```python
from build123d import *

# Parameters (mm, degrees)
BOSS_EXTRUDE1_DEPTH = 5.08
SKETCH4_R           = 104.775
CUT_EXTRUDE1_DEPTH  = 50.8
SKETCH5_R           = 3.175
CUT_EXTRUDE2_DEPTH  = 5.08
SKETCH6_R           = 3.175
CUT_EXTRUDE3_DEPTH  = 5.08


with BuildPart() as part:
    # Sketch2 → Boss-Extrude1 (new body)
    with BuildSketch(Plane(origin=(0, 0, 0), x_dir=(1, 0, 0), z_dir=(0, 1, 0))):
        Polygon((-203.2, 381), (-44.423028516, 381), (-44.423028516, 423.747508854), (44.020558762, 423.747508854), (44.020558762, 381), (381, 381), (381, 0), (-203.2, 0), align=None)
    extrude(amount=BOSS_EXTRUDE1_DEPTH)

    # Sketch4 → Cut-Extrude1 (cut)
    with BuildSketch(Plane.XZ):
        with Locations((0, -381)):
            Circle(SKETCH4_R)
    extrude(amount=-CUT_EXTRUDE1_DEPTH, mode=Mode.SUBTRACT)

    # Sketch5 → Cut-Extrude2 (cut)
    with BuildSketch(Plane(origin=(0, 5.08, 0), x_dir=(1, 0, 0), z_dir=(0, 1, 0))):
        with Locations(Location((332.74, 177.8, 0), (0, 0, 270))):
            Circle(SKETCH5_R)
        with Locations(Location((101.6, 6.35, 0), (0, 0, 270))):
            Circle(SKETCH5_R)
        with Locations(Location((203.2, 48.26, 0), (0, 0, 270))):
            Circle(SKETCH5_R)
        with Locations(Location((279.4, 101.6, 0), (0, 0, 270))):
            Circle(SKETCH5_R)
        with Locations(Location((368.3, 152.4, 0), (0, 0, 270))):
            Circle(SKETCH5_R)
        with Locations(Location((374.65, 279.4, 0), (0, 0, 270))):
            Circle(SKETCH5_R)
        with Locations(Location((368.3, 12.7, 0), (0, 0, 270))):
            Circle(SKETCH5_R)
        with Locations(Location((228.6, 12.7, 0), (0, 0, 270))):
            Circle(SKETCH5_R)
    extrude(amount=-CUT_EXTRUDE2_DEPTH, mode=Mode.SUBTRACT)

    # Sketch6 → Cut-Extrude3 (cut)
    with BuildSketch(Plane(origin=(0, 5.08, 0), x_dir=(1, 0, 0), z_dir=(0, 1, 0))):
        with Locations(Location((-190.5, 368.3, 0), (0, 0, 270))):
            Circle(SKETCH6_R)
        with Locations(Location((-116.84, 368.3, 0), (0, 0, 270))):
            Circle(SKETCH6_R)
        with Locations(Location((-83.82, 302.26, 0), (0, 0, 270))):
            Circle(SKETCH6_R)
        with Locations(Location((-142.24, 281.94, 0), (0, 0, 270))):
            Circle(SKETCH6_R)
        with Locations(Location((-190.5, 233.68, 0), (0, 0, 270))):
            Circle(SKETCH6_R)
        with Locations(Location((-190.5, 304.8, 0), (0, 0, 270))):
            Circle(SKETCH6_R)
    extrude(amount=-CUT_EXTRUDE3_DEPTH, mode=Mode.SUBTRACT)


solid = part.part
```
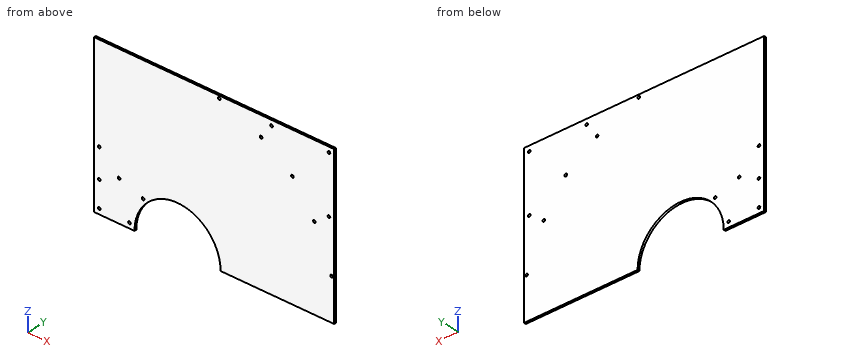
Work out the finished part from the listing and answer in its coordinate system (mm). Coordinates: 2 decimals unless noted, no trailing zeros. Loops run counter-clockwise (first coordinate to the right, second up) from the corner with the lowest first, then second, coordinate; pieces in that order, holes last. Notation, with made-up numbers: (-33, 3) - (-2, 3) arc R31 cw to (-2, 31) - close; hole circle Ø3 at (13, -15.75). An arc over 180 degrees is marked (long way). Use a Markdown table: item, result.
Item 1: Find section C-C, the plane x = 90.5. Determine the outline of the cut face in (y, z), and give its area (3 significant figures).
Evaluation:
| item | result |
|---|---|
| outline | (0, -328.2) - (5.08, -328.2) - (5.08, 0) - (0, 0) - close |
| area | 1,670 mm2 |
Item 2: Consider probe 1 along Z at (x, y) = (-190.5, 1.75) (3 decimals); probe 2 along Z at (x, y) = (332.74, 2.7) (3 decimals); probe 3 along X at (y, z) = (3.5, -233.68) (3 decimals). Determine where each line is inside the solid, lowest interval first. Write a range as from..to.
Evaluation:
| item | result |
|---|---|
| probe 1 | z = -381..-371.475, -365.125..-307.975, -301.625..-236.855, -230.505..0 |
| probe 2 | z = -381..-180.975, -174.625..0 |
| probe 3 | x = -203.2..-193.675, -187.325..381 |
Item 3: Find section B-B, the plane y = 0.8. State how many separate pieces and enclosed holes the cut face has, and give its area (3 significant figures).
Evaluation:
| item | result |
|---|---|
| separate pieces | 1 |
| enclosed holes | 14 |
| area | 205,000 mm2 |
Item 4: Find section A-A, the plane z = -349. Determine the outline of the cut face in (x, y).
Evaluation:
| item | result |
|---|---|
| outline | (-203.2, 0) - (-99.77, 0) - (-99.77, 5.08) - (-203.2, 5.08) - close; (99.77, 0) - (381, 0) - (381, 5.08) - (99.77, 5.08) - close |
